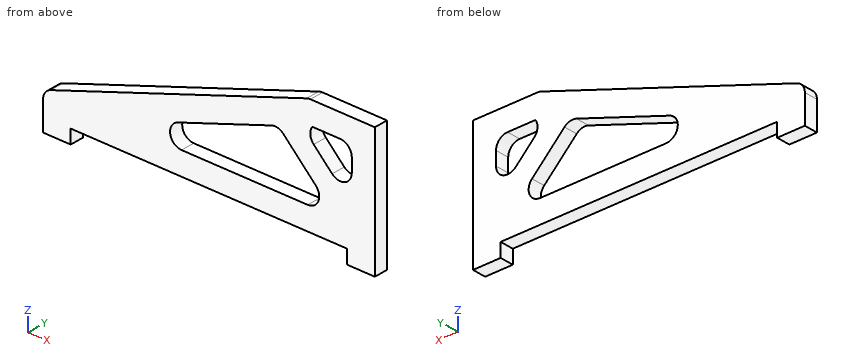
from build123d import *

# Parameters (mm, degrees)
SKETCH1_W           = 6
SKETCH1_H           = 3
BOSS_EXTRUDE1_DEPTH = 3
CUT_EXTRUDE1_REACH  = 41.31
FILLET1_R           = 2.5


with BuildPart() as part:
    # Sketch1 → Boss-Extrude1 (new body)
    with BuildSketch(Plane(origin=(0, 0, 0), x_dir=(1, 0, 0), z_dir=(0, 1, 0))):
        Polygon((-36, 12.5), (-36, 7.5), (21.6, -12.5), (36, -12.5), (36, 12.5), (30, 12.5), (-30, 12.5), align=None)
        with Locations((-33, 14)):
            Rectangle(SKETCH1_W, SKETCH1_H)
        with Locations((33, 14)):
            Rectangle(SKETCH1_W, SKETCH1_H)
    extrude(amount=BOSS_EXTRUDE1_DEPTH)

    # Sketch2 → Cut-Extrude1 (cut, up to next)
    with BuildSketch(Plane(origin=(0, 3, 0), x_dir=(1, 0, 0), z_dir=(0, 1, 0)), mode=Mode.PRIVATE) as cut_extrude1_sk1:
        Polygon((-20.75664079, 7.5), (15.036345763, -4.928120331), (27.464466094, 7.5), align=None)
    cut_extrude1_tool1 = extrude(cut_extrude1_sk1.sketch, amount=-CUT_EXTRUDE1_REACH, mode=Mode.PRIVATE) & part.part
    # Sketch2 → Cut-Extrude1 (cut, up to next)
    with BuildSketch(Plane(origin=(0, 3, 0), x_dir=(1, 0, 0), z_dir=(0, 1, 0)), mode=Mode.PRIVATE) as cut_extrude1_sk2:
        Polygon((31, 3.964466094), (20.284973417, -6.750560489), (22.44335921, -7.5), (31, -7.5), align=None)
    cut_extrude1_tool2 = extrude(cut_extrude1_sk2.sketch, amount=-CUT_EXTRUDE1_REACH, mode=Mode.PRIVATE) & part.part
    add(cut_extrude1_tool1.solids().sort_by_distance((7.248057, 3, -3.357293))[0], mode=Mode.SUBTRACT)
    add(cut_extrude1_tool2.solids().sort_by_distance((27.286818, 3, 3.618293))[0], mode=Mode.SUBTRACT)

    # Fillet1
    # the kernel refuses this fillet: 2.5 mm, written as the material it adds along each edge
    with BuildSketch(Plane(origin=(20.284973417, 3, 6.750560489), x_dir=(0.7071067811865467, 0, -0.7071067811865482), z_dir=(0, -1, 0))) as fillet1_piece_1:
        with BuildLine():
            CenterArc((3.456558168, 2.5), FILLET1_R, 190.226667661, 79.773332339)
            Line((0.99627547, 2.056142991), (0, 0))
            Line((0, 0), (3.456558168, 0))
        make_face()
    extrude(amount=3)
    with BuildSketch(Plane(origin=(31, 3, -3.964466094), x_dir=(0, 0, 1), z_dir=(0, -1, 0)), Plane(origin=(27.464466094, 3, -7.5), x_dir=(-0.7071067811865461, 0, 0.707106781186549), z_dir=(0, -1, 0))) as fillet1_piece_2:
        with BuildLine():
            CenterArc((FILLET1_R * 2.41421356237, FILLET1_R), FILLET1_R, 135, 135)
            Line((FILLET1_R * 1.70710678119, FILLET1_R * 1.70710678119), (0, 0))
            Line((0, 0), (FILLET1_R * 2.41421356237, 0))
        make_face()
    extrude(amount=3)
    with BuildSketch(Plane(origin=(31, 3, 7.5), x_dir=(0, 0, -1), z_dir=(0, -1, 0))) as fillet1_piece_3:
        with BuildLine():
            CenterArc((FILLET1_R, -FILLET1_R), FILLET1_R, 90, 90)
            Line((0, -FILLET1_R), (0, 0))
            Line((0, 0), (FILLET1_R, 0))
        make_face()
    extrude(amount=3)
    with BuildSketch(Plane(origin=(-20.75664079, 3, -7.5), x_dir=(0.9446736642347862, 0, 0.3280116889704124), z_dir=(0, -1, 0))) as fillet1_piece_4:
        with BuildLine():
            CenterArc((FILLET1_R * 5.92867184197, -FILLET1_R), FILLET1_R, 90, 160.851862542)
            Line((FILLET1_R * 5.600660153, -FILLET1_R * 1.94467366423), (0, 0))
            Line((0, 0), (FILLET1_R * 5.92867184197, 0))
        make_face()
    extrude(amount=3)
    with BuildSketch(Plane(origin=(15.036345763, 3, 4.928120331), x_dir=(-0.9446736642347863, 0, -0.3280116889704122), z_dir=(0, -1, 0))) as fillet1_piece_5:
        with BuildLine():
            CenterArc((FILLET1_R * 0.626668316014, FILLET1_R), FILLET1_R, 205.851862542, 64.148137458)
            Line((-FILLET1_R * 0.273256127554, FILLET1_R * 0.563954135591), (0, 0))
            Line((0, 0), (FILLET1_R * 0.626668316014, 0))
        make_face()
    extrude(amount=3)
    # the kernel refuses this fillet: 2.5 mm, written as the material it takes off along each edge
    with BuildSketch(Plane(origin=(21.6, -1.054199012, 12.5), x_dir=(-0.9446736642347879, 0, -0.32801168897040733), z_dir=(0, 1, 0))) as fillet1_2_piece_1:
        with BuildLine():
            CenterArc((FILLET1_R * 0.168671841967, -FILLET1_R), FILLET1_R, 90, 19.148137458)
            Line((-FILLET1_R * 0.159339847004, -FILLET1_R * 0.0553263357652), (0, 0))
            Line((0, 0), (FILLET1_R * 0.168671841967, 0))
        make_face()
    extrude(amount=5.108398025, mode=Mode.SUBTRACT)
    with BuildSketch(Plane(origin=(-36, -4.445902435, -7.5), x_dir=(0, 0, -1), z_dir=(0, 1, 0))) as fillet1_2_piece_2:
        with BuildLine():
            CenterArc((FILLET1_R * 0.711344389572, -FILLET1_R), FILLET1_R, 90, 70.851862542)
            Line((-FILLET1_R * 0.233329274663, -FILLET1_R * 0.67198831103), (0, 0))
            Line((0, 0), (FILLET1_R * 0.711344389572, 0))
        make_face()
    extrude(amount=11.89180487, mode=Mode.SUBTRACT)


solid = part.part
Part model, mm, in its own coordinate system. Give positions to 0.01 mm unless a question says otherwise; leave off trailing zeros. Loops run counter-clockwise (first coordinate to the right, second up) from the corner with the lowest first, then second, coordinate; pieces in that order, holes last.
(1) Band-saw the part on B-B (x = 18.5). Write the cut outline in (y, z), and give its area (3 significant figures).
Return value:
outline: (0, -12.5) - (3, -12.5) - (3, -7.5) - (0, -7.5) - close; (0, 1.46) - (3, 1.46) - (3, 11.42) - (0, 11.42) - close
area: 44.9 mm2
(2) Band-saw the part on A-A (y = 1.1). Write the cut outline in (x, z) (3 decimals).
Return value:
outline: (-36, -15.5) - (-30, -15.5) - (-30, -12.5) - (30, -12.5) - (30, -15.5) - (36, -15.5) - (36, 12.5) - (22.022, 12.5) arc R2.5 ccw to (21.202, 12.362) - (-34.32, -6.917) arc R2.5 ccw to (-36, -9.278) - close; hole (-6.755, -2.638) arc R2.5 ccw to (-5.935, -7.5) - (21.429, -7.5) arc R2.5 ccw to (23.197, -3.232) - (16.144, 3.82) arc R2.5 ccw to (13.556, 4.414) - close; hole (22.443, 7.5) arc R2.5 ccw to (22.729, 4.306) - (26.732, 0.303) arc R2.5 ccw to (31, 2.071) - (31, 5) arc R2.5 ccw to (28.5, 7.5) - close
(3) Band-saw the part on D-D (z = 8.75). Write the cut outline in (x, y), and give its area (3 significant figures).
Return value:
outline: (10.8, 0) - (36, 0) - (36, 3) - (10.8, 3) - close
area: 75.6 mm2
(4) Pin check, flat tip, straight feed: pin 1 (1.5 mm diameter, centred on x = 25.5, y = 2, fed in from -Z). Stop position of the tip, or through.
Return value:
pin 1: stops at z = -12.5
(5) Band-saw the part on C-C (z = -1.5). Write the cut outline in (x, y), and give its area (3 significant figures).
Return value:
outline: (-18.72, 0) - (-3.48, 0) - (-3.48, 3) - (-18.72, 3) - close; (21.46, 0) - (36, 0) - (36, 3) - (21.46, 3) - close
area: 89.3 mm2
(6) Drill centre lines: line 1 along Z through (x, y) = (1.5, 1.7); line 2 along X through (y, z) = (1.2, -14); line 3 along Z through (x, y) = (-7.5, 0.7). Where is each one in solid material? Low to high.
Return value:
line 1: z = -12.5 to -7.5, 0.23 to 5.52
line 2: x = -36 to -30, 30 to 36
line 3: z = -12.5 to -6.95, -3.05 to 2.4
